from build123d import *

# Parameters (mm, degrees)
F0_W     = 60.8292
F0_H     = 71.166755
F1_DEPTH = 3.175
F0_W_2   = 2.54
F0_H_2   = 38.1
F2_DEPTH = 3.175


with BuildPart() as f1:
    # F0 (on Top) → F1 (new body)
    with BuildSketch(Plane.XY):
        Polygon((0, 94.343368), (0, 0.757935), (60.8292, 0.757935), (20.6375, 132.443368), (2.54, 132.443368), (2.54, 94.343368), align=None)
        Polygon((-2.54, 132.443368), (-20.6375, 132.443368), (-60.8292, 0.757935), (0, 0.757935), (0, 94.343368), (-2.54, 94.343368), align=None)
        with Locations((-30.4146, -34.825442)):
            Rectangle(F0_W, F0_H)
        with Locations((30.4146, -34.825442)):
            Rectangle(F0_W, F0_H)
    extrude(amount=F1_DEPTH)

    # F0 (on Top) → F2 (cut)
    with BuildSketch(Plane.XY):
        with Locations((-1.27, 113.393368)):
            Rectangle(F0_W_2, F0_H_2)
        with Locations((1.27, 113.393368)):
            Rectangle(F0_W_2, F0_H_2)
    extrude(amount=-F2_DEPTH, mode=Mode.SUBTRACT)


solid = f1.part
Verification items for the finished model (mm, model axes). Coordinates: 2 decimals unless noted, no trailing zeros. Order: outer loops, then holes, each group sorted by start corner. A loop starts at its lowest first (then second) coordinate and runs counter-clockwise, first axis right, second up. Notation, with made-up numbers: (-24.75, 80.25) -> (14.25, 80.25) arc R31 cw to (14.25, 117.25) -> close; hole circle Ø8 at (12, 58). An arc over 180 degrees is marked (long way). Put each result on its own line as item: value. Start each with the question number.
1. Material ranges on L1, parallel to X at y = 117.5, z = 2.5; L2, parallel to X at y = 65.5, z = 1.3; L3, parallel to X at y = 58, z = 1.1, recorded low to high. Write a range as [from, to].
2. Cross-section at C-C, the plane y = 69.5. Record the boundary of the cut face in (x, z) (3 decimals).
3. Cross-section at A-A, the plane z = 1.3. Record the boundary of the cut face in (x, y).
4. Cross-section at B-B, the plane x = 46. Record the boundary of the cut face in (y, z) (3 decimals), then the cut area to 3 significant figures.
5. Go/stop test with flat-tipped pins: pin 1 Ø1 at (y, z) = (106.5, 1.5) entering from +X; pin 2 Ø8 at (x, y) = (35, 18.5) entering from -Z; pin 3 Ø1 at (y, z) = (33.5, 1) entering from +X. Record where each tip stops, or that it passes through.
6. Mould release check, pull along X, two halves, no side actions. Record for faces 1 (the flat face through (-1, 10, 3.175)), 2 (the flat face through (-40.452, 67.522, 1.565)), 3 (the flat face through (41.015, 65.679, 1.565)): released by +X, released by -X, zero draft, split by the parting line, or undercut.
Computed:
1. L1: [-25.2, -2.54], [2.54, 25.2]
1. L2: [-41.07, 41.07]
1. L3: [-43.36, 43.36]
2. outline: (-39.848, 0) -> (39.848, 0) -> (39.848, 3.175) -> (-39.848, 3.175) -> close
3. outline: (-60.83, -70.41) -> (60.83, -70.41) -> (60.83, 0.76) -> (20.64, 132.44) -> (2.54, 132.44) -> (2.54, 94.34) -> (-2.54, 94.34) -> (-2.54, 132.44) -> (-20.64, 132.44) -> (-60.83, 0.76) -> close
4. outline: (-70.409, 0) -> (49.345, 0) -> (49.345, 3.175) -> (-70.409, 3.175) -> close
4. area: 380 mm2
5. pin 1: x = 28.71
5. pin 2: z = 0
5. pin 3: x = 50.99
6. face 1: zero draft
6. face 2: released by -X
6. face 3: released by +X
